Geometry: final body of the model. Coordinates: model frame, mm. A direction names the side the tool comes from. Coordinates: 2 decimals unless noted, no trailing zeros. Write each loop counter-clockwise with the first axis right and the second up, starting at its lowest first coordinate (ties: lowest second). Pieces come first, ordered by that corner, then holes. Notation, with made-up numbers: (50.5, 13) - (58.5, 13) arc R12 cw to (58.5, 23) - close; hole circle Ø9 at (48.5, -17). An arc over 180 degrees is marked (long way). Put each result on its own line as item: value.
```python
from build123d import *

# Parameters (mm, degrees)
SKETCH1_R          = 15
STOCK_DEPTH        = 29.75
HEX_HEAD_DEPTH     = 8.5
SKETCH5_R          = 14
RETAINER_DEPTH     = 2.5
SKETCH9_W          = 1.368260999
SKETCH9_H          = 3.99
SKETCH9_W_2        = 1.545391276
CUT_EXTRUDE3_DEPTH = 13.475
SKETCH10_R         = 5.98
EXTRUDE4_DEPTH     = 11.01
SKETCH11_R         = 5.98
SKETCH11_R_2       = 5.775
CUT_EXTRUDE4_DEPTH = 5
SKETCH13_W         = 0.98
SKETCH13_H         = 5
CUT_EXTRUDE5_DEPTH = 15


with BuildPart() as part:
    # Sketch1 → STOCK (new body, symmetric)
    with BuildSketch(Plane(origin=(0, 0, 0), x_dir=(1, 0, 0), z_dir=(0, 1, 0))):
        with Locations(Location((0, 0, 0), (0, 0, 270))):  # turned: the seam where the file's is
            Circle(SKETCH1_R)
    extrude(amount=STOCK_DEPTH, both=True)

    # Sketch2 → HEX_HEAD (cut)
    with BuildSketch(Plane(origin=(0, 29.75, 0), x_dir=(1, 0, 0), z_dir=(0, 1, 0))):
        with BuildLine():
            ThreePointArc((12.412375826, 8.422168743), (7.5, 12.990381057), (1.087624174, 14.960517159))
            Line((1.087624174, 14.960517159), (12.412375826, 8.422168743))
        make_face()
        with BuildLine():
            Line((-12.412375826, 8.422168743), (-1.087624174, 14.960517159))
            ThreePointArc((-1.087624174, 14.960517159), (-7.5, 12.990381057), (-12.412375826, 8.422168743))
        make_face()
        with BuildLine():
            Line((13.5, 6.538348415), (13.5, -6.538348415))
            ThreePointArc((13.5, -6.538348415), (15, 0), (13.5, 6.538348415))
        make_face()
        with BuildLine():
            Line((-13.5, -6.538348415), (-13.5, 6.538348415))
            ThreePointArc((-13.5, 6.538348415), (-15, 0), (-13.5, -6.538348415))
        make_face()
        with BuildLine():
            Line((12.412375826, -8.422168743), (1.087624174, -14.960517159))
            ThreePointArc((1.087624174, -14.960517159), (7.5, -12.990381057), (12.412375826, -8.422168743))
        make_face()
        with BuildLine():
            Line((-1.087624174, -14.960517159), (-12.412375826, -8.422168743))
            ThreePointArc((-12.412375826, -8.422168743), (-7.5, -12.990381057), (-1.087624174, -14.960517159))
        make_face()
    extrude(amount=-HEX_HEAD_DEPTH, mode=Mode.SUBTRACT)

    # Sketch3 → CROWN (revolve, cut)
    with BuildSketch(Plane.XY, mode=Mode.PRIVATE) as crown_sk:
        Polygon((10.25, 29.75), (15, 29.75), (15, 28.477241336), align=None)
    revolve(crown_sk.sketch.rotate(Axis((0, 0, 0), (0, 1, 0)), 94.158067237), axis=Axis((0, 0, 0), (0, 1, 0)), mode=Mode.SUBTRACT)  # turned: the seam where the file's is

    # Sketch4 → Cut-Revolve1 (revolve, cut)
    with BuildSketch(Plane.XY, mode=Mode.PRIVATE) as cut_revolve1_sk:
        Polygon((14.125, -29.75), (16.897307641, -29.75), (16.897307641, 25.522307641), (13.875, 22.5), (13.875, 21), (14.925, 19.95), (14.925, -22.04), (14.125, -22.84), align=None)
    revolve(cut_revolve1_sk.sketch.rotate(Axis((0, -34.538461529, 0), (0, 1, 0)), 90), axis=Axis((0, -34.538461529, 0), (0, 1, 0)), mode=Mode.SUBTRACT)  # turned: the seam where the file's is

    # Sketch5 → RETAINER (add)
    with BuildSketch(Plane.XZ.offset(29.75)):
        with Locations(Location((0, 0, 0), (0, 0, 90))):  # turned: the seam where the file's is
            Circle(SKETCH5_R)
    extrude(amount=RETAINER_DEPTH)



with BuildPart() as body_2:
    # Sketch8 → Revolve1 (revolve)
    with BuildSketch(Plane.XY, mode=Mode.PRIVATE) as revolve1_sk:
        Polygon((0, 44.75), (4, 44.75), (5.75, 43), (5.75, 40.76), (0, 40.76), align=None)
    revolve(revolve1_sk.sketch.rotate(Axis((0, 0, 0), (0, 1, 0)), 90), axis=Axis((0, 0, 0), (0, 1, 0)))  # turned: the seam where the file's is

    # Sketch9 → Cut-Extrude3 (cut, symmetric)
    with BuildSketch(Plane.XY):
        with Locations((5.6841305, 42.755)):
            Rectangle(SKETCH9_W, SKETCH9_H)
        with Locations((-5.772695638, 42.755)):
            Rectangle(SKETCH9_W_2, SKETCH9_H)
    extrude(amount=CUT_EXTRUDE3_DEPTH, both=True, mode=Mode.SUBTRACT)


with BuildPart() as part_1:
    add(part.part)

    add(body_2.part)  # Extrude4 merges body 2
    # Sketch10 → Extrude4 (add)
    with BuildSketch(Plane(origin=(0, 29.75, 0), x_dir=(1, 0, 0), z_dir=(0, 1, 0))):
        with Locations(Location((0, 0, 0), (0, 0, 180))):  # turned: the seam where the file's is
            Circle(SKETCH10_R)
    extrude(amount=EXTRUDE4_DEPTH)

    # Sketch11 → Cut-Extrude4 (cut)
    with BuildSketch(Plane(origin=(0, 40.76, 0), x_dir=(1, 0, 0), z_dir=(0, 1, 0))):
        with Locations(Location((0, 0, 0), (0, 0, 180))):  # turned: the seam where the file's is
            Circle(SKETCH11_R)
        with Locations(Location((0, 0, 0), (0, 0, 180))):  # turned: the seam where the file's is
            Circle(SKETCH11_R_2, mode=Mode.SUBTRACT)
    extrude(amount=-CUT_EXTRUDE4_DEPTH, mode=Mode.SUBTRACT)

    # Sketch13 → Cut-Extrude5 (cut, symmetric)
    with BuildSketch(Plane.XY):
        with Locations((5.49, 38.26)):
            Rectangle(SKETCH13_W, SKETCH13_H)
        with Locations((-5.49, 38.26)):
            Rectangle(SKETCH13_W, SKETCH13_H)
    extrude(amount=CUT_EXTRUDE5_DEPTH, both=True, mode=Mode.SUBTRACT)


solid = part_1.part
```
1. Ray query, probe 1 along Y at (x, z) = (1, -10); probe 2 along X at (y, z) = (19, 0) (3 decimals); probe 3 along X at (y, z) = (-12, 11). Return the intervals inside material, ascending. Write a range as from..to.
Answer below:
probe 1: y = -32.25..29.75
probe 2: x = -14.925..14.925
probe 3: x = -10.09..10.09
2. Set-up query: faces 4 (the flat face through (5, 40, 0)), 5 (the cylindrical face through (0.08, 41.86, -5.75)), 6 (the flat face through (-5.3, 35.76, 0.5)), 7 (the cylindrical face through (13.67, -30.98, -3.03)), 8 (the flat face through (6.671, 25.118, -11.737)). Return all of +Z, -Z, +X, -X, +Y, -Y with unobstructed straight access to the full face (end or side cutting, diameter ignored); none if empty.
Answer below:
face 4: +Z, -Z, +X, +Y
face 5: -Z, +Y
face 6: +Y
face 7: -Y
face 8: -Z, +X, +Y
3. Mould query, pull axis Y, two halves, no side actions, for faces 1 (the conical face through (-12.42, 22.93, 7.1)), 2 (the flat face through (-6.8, 21.25, 11.9)), 3 (the flat face through (13.5, 25, 0)). Classes: +Y half, -Y half, draft (parallel to the pull), parting line (faces both ways), or undercut.
Answer below:
face 1: undercut
face 2: +Y half
face 3: draft
4. Section query B-B (y = 8). Return loops of the section in (x, z) (3 decimals), then the cut area to 3 significant figures.
Answer below:
outline: circle Ø29.85 at (0, 0)
area: 700 mm²
5. Pin query (flat end, axial travel): pin 1 Ø4 at (y, z) = (-21, -10) entering from -X; pin 2 Ø2.5 at (x, z) = (-7.5, -11) entering from +Y; pin 3 Ø0.9 at (x, z) = (-2, -4.5) entering from +Y. Return the tip coordinate at first contact, or that it passes through.
Answer below:
pin 1: stops at x = -12.6
pin 2: stops at y = 29.26
pin 3: stops at y = 44.28
